Geometry check sheet. Reference: the model listing, model coordinates, mm. Face numbers are marked on the shaded views. A direction names the side the tool comes from. Round coordinates to 2 decimals unless told otherwise and drop trailing zeros. Order: outer loops, then holes, each group sorted by start corner. A loop starts at its lowest first (then second) coordinate and runs counter-clockwise, first axis right, second up. Notation, with made-up numbers: (46, 19.25) -> (76, 19.25) arc R18 ccw to (76, 43.25) -> close; hole circle Ø10 at (2, 24). An arc over 180 degrees is marked (long way). Use a Markdown table: item, result. Add a question column.
Item 1: Set-up check for the marked faces 4, 5 and 6: record each of +Z, -Z, +X, -X, +Y, -Y from which the full face is reachable in a straight line by a thin tool's end or side.
Item 2: Sectioned sample at D-D, the plane x = -2.25. Record the cut outline in (y, z), and give its area (3 significant figures).
Item 3: Material ranges on probe 1 along Z at (x, y) = (0.79, 4); probe 2 along Y at (x, z) = (4.25, 0); probe 3 along X at (y, z) = (1, -0.75), recorded low to high. Write a range as [from, to].
Item 4: Mould release check, pull along X, two halves, no side actions. Record for the marked faces 1, 2 and 3: pulls with the +X half, pulls with the -X half, needs draft (parallel to the pull), parting line crosses it, or undercut.
Item 5: Gauge pin test, flat end, axial feed: pin 1 Ø1 at (y, z) = (2.5, 0) entering from +X. Record the tip position at first contact, or that the pin passes through.
Item 6: Sectioned sample at B-B, the plane y = 1. Record the cut outline in (x, z).
Item 7: Sectioned sample at A-A, the plane z = 0. Record the cut outline in (x, y) (3 decimals), and give its area (3 significant figures).
Item 8: Sectioned sample at C-C, the plane x = 1.5. Record the cut outline in (y, z), and give its area (3 significant figures).
Autodesk Inventor part; units mm, degrees
ref_plane "YZ Plane" through (0, 0, 0) normal (1, 0, 0) x (0, 1, 0)
ref_plane "XZ Plane" through (0, 0, 0) normal (0, 1, 0) x (-1, 0, 0)
ref_plane "XY Plane" through (0, 0, 0) normal (0, 0, 1) x (1, 0, 0)
sketch "Sketch1" plane through (0, 0, 0) normal (0, 1, 0) x (-1, 0, 0)
  line L0 (-4.567, 3.1368) -> (-0.433, 5.5235)
  line L1 (0.433, 5.5235) -> (4.567, 3.1368)
  line L2 (5, 2.3868) -> (5, -2.3868)
  line L3 (4.567, -3.1368) -> (0.433, -5.5235)
  line L4 (-0.433, -5.5235) -> (-4.567, -3.1368)
  circle A0 centre (0, 0) radius 3.555
  circle A1 centre (-0.79, 0) radius 2.5
  line L5 (0.433, 5.5235) -> (-0.433, 5.5235)
  line L6 (-4.567, 3.1368) -> (-5, 2.3868)
  line L7 (4.567, 3.1368) -> (5, 2.3868)
  line L8 (5, -2.3868) -> (4.567, -3.1368)
  line L9 (0.433, -5.5235) -> (-0.433, -5.5235)
  line L10 (-4.567, -3.1368) -> (-5, -2.3868)
  line L11 (-5, -1) -> (-4.85, -1)
  line L12 (-4.85, -1) -> (-4.85, 1)
  line L13 (-4.85, 1) -> (-5, 1)
  line L14 (-5, -2.3868) -> (-5, -1)
  line L15 (-5, 1) -> (-5, 2.3868)
  point P0 (-5, 2.8868)
  point P1 (0, 5.7735)
  point P2 (5, 2.8868)
  point P3 (5, -2.8868)
  point P4 (0, -5.7735)
  point P5 (-5, -2.8868)
  point P6 (-4.85, 0)
  dimension "d1" = 7.11
  dimension "d2" = 5
  dimension "d3" = 0.79
  dimension "d4" = 0.5
  dimension "d5" = 0.5
  dimension "d6" = 0.5
  dimension "d7" = 0.5
  dimension "d8" = 0.5
  dimension "d9" = 0.5
  dimension "d10" = 0.5
  dimension "d11" = 0.5
  dimension "d12" = 0.5
  dimension "d13" = 0.5
  dimension "d14" = 0.5
  dimension "d15" = 0.5
  dimension "d16" = 2
extrude "Extrusion1" add sketch "Sketch1" along normal blind 6 contours L0 L5 L1 L7 L2 L8 L3 L9 L4 L10 L14 L11 L12 L13 L15 L6 | A0
extrude "Extrusion2" add sketch "Sketch1" against normal blind 2.5 contours A0
chamfer "Chamfer1" distance 0.5 angle 45 12 edges at (-4.7835, 0, -2.7618) (0, 0, -5.5235) (-4.7835, 0, 2.7618) (4.7835, 0, -2.7618) (4.7835, 0, 2.7618) (0, 0, 5.5235) (4.7835, 6, 2.7618) (0, 6, 5.5235) (-4.7835, 6, 2.7618) (-4.7835, 6, -2.7618) (0, 6, -5.5235) (4.7835, 6, -2.7618)
properties part number "Eccentric Spacer"
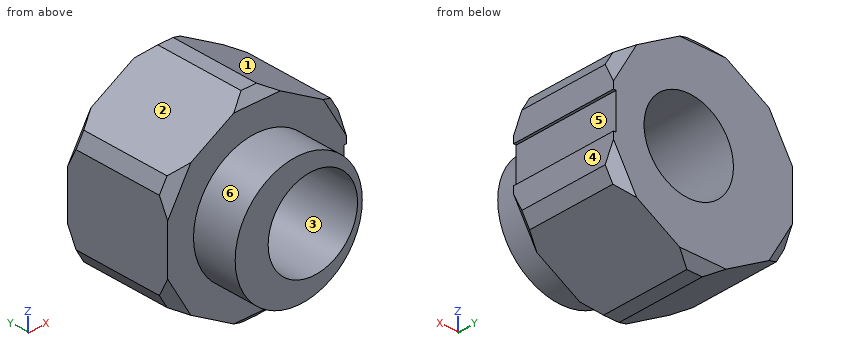
Found:
| question | item | result |
|---|---|---|
| 1 | face 4 | +Z, -Z, +X, +Y, -Y |
| 1 | face 5 | +X, +Y, -Y |
| 1 | face 6 | -Y |
| 2 | outline | (-2.5, -2.75) -> (0, -2.75) -> (0, -4.47) -> (6, -4.47) -> (6, 4.47) -> (0, 4.47) -> (0, 2.75) -> (-2.5, 2.75) -> close |
| 2 | area | 67.5 mm2 |
| 3 | probe 1 | z = [-5.32, -2.5], [2.5, 5.32] |
| 3 | probe 2 | y = [0, 6] |
| 3 | probe 3 | x = [-5, -1.59], [3.17, 4.85] |
| 4 | face 1 | pulls with the +X half |
| 4 | face 2 | pulls with the -X half |
| 4 | face 3 | undercut |
| 5 | pin 1 | stops at x = 4.85 |
| 6 | outline | (-5, -2.39) -> (-4.57, -3.14) -> (-0.43, -5.52) -> (0.43, -5.52) -> (4.57, -3.14) -> (5, -2.39) -> (5, -1) -> (4.85, -1) -> (4.85, 1) -> (5, 1) -> (5, 2.39) -> (4.57, 3.14) -> (0.43, 5.52) -> (-0.43, 5.52) -> (-4.57, 3.14) -> (-5, 2.39) -> close; hole circle Ø5 at (0.79, 0) |
| 7 | outline | (-5, 0) -> (-3.555, 0) -> (-3.555, -2.5) -> (-1.71, -2.5) -> (-1.71, 6) -> (-5, 6) -> close; (3.29, -2.5) -> (3.555, -2.5) -> (3.555, 0) -> (4.85, 0) -> (4.85, 6) -> (3.29, 6) -> close |
| 7 | area | 34.4 mm2 |
| 8 | outline | (-2.5, -3.22) -> (0, -3.22) -> (0, -4.91) -> (6, -4.91) -> (6, -2.4) -> (-2.5, -2.4) -> close; (-2.5, 2.4) -> (6, 2.4) -> (6, 4.91) -> (0, 4.91) -> (0, 3.22) -> (-2.5, 3.22) -> close |
| 8 | area | 34.3 mm2 |
